Geometry: final body of the model. Coordinates: model frame, mm. Round coordinates to 2 decimals unless told otherwise and drop trailing zeros. Return JSON: item names as keys, results as strings. Group by question number.
Q1. Ray query, probe 1 along Y at (x, z) = (5.75, 0); probe 2 along Y at (x, z) = (5.5, -26.5); probe 3 along Z at (x, y) = (6.75, -94). Return the intervals inside material, ascending.
Q2. Mould query, pull axis Y, two halves, no side actions, for faces 1 (the face through (8, -32, 2)), 2 (the face through (4.06, 44.86, 39.25)), 3 (the face through (3.948, 154.672, 20.308)). Classes: released by +Y, released by -Y, zero draft, split by the parting line, or undercut.
Q3. Cut plane A-A on x = 4.25. Count the separate pieces of the cut face and the enclosed holes in it, and give its area (3 significant figures).
Q4. Contact query for flat-ended pins moving along their axis: pin 1 (6.5 mm diameter, centred on y = 42.43, z = 42.43, fed in from +X); pin 2 (3 mm diameter, centred on x = 3, y = 50, fed in from -Z); pin 3 (1 mm diameter, centred on x = 4.5, z = -58.5, fed in from +Y); pin 4 (3 mm diameter, centred on x = 7, z = 45, fed in from +Y). Output: stop coordinate, or through.
```python
from build123d import *

# Parameters (mm, degrees)
SKETCH_1_R               = 156
EXTRUDE_1_DEPTH          = 8
SKETCH_2_R               = 31
CUT_EXTRUDE_1_DEPTH      = 10
SKETCH_4_R               = 6
CUT_EXTRUDE_3_DEPTH      = 10
PATTERN_CIRCULAR_2_COUNT = 4
SKETCH_6_R               = 2
CUT_EXTRUDE_5_DEPTH      = 10
PATTERN_CIRCULAR_4_COUNT = 4
FILLET_1_R               = 0.3
SKETCH_8_R               = 4
CUT_EXTRUDE_7_DEPTH      = 10
SKETCH_9_R               = 30
CUT_EXTRUDE_8_DEPTH      = 10
PATTERN_CIRCULAR_6_COUNT = 4
PATTERN_CIRCULAR_7_COUNT = 2


with BuildPart() as part:
    # 草图1 → 凸台-拉伸1 (new body)
    with BuildSketch(Plane(origin=(0, 0, 0), x_dir=(0, 0, -1), z_dir=(1, 0, 0))):
        Circle(SKETCH_1_R)
    extrude(amount=EXTRUDE_1_DEPTH)

    # 草图2 → 切除-拉伸1 (cut)
    with BuildSketch(Plane(origin=(8, 0, 0), x_dir=(0, 0, -1), z_dir=(1, 0, 0))):
        Circle(SKETCH_2_R)
    extrude(amount=-CUT_EXTRUDE_1_DEPTH, mode=Mode.SUBTRACT)

    # 草图4 → 切除-拉伸3 (cut)
    with BuildSketch(Plane(origin=(8, 0, 0), x_dir=(0, 0, -1), z_dir=(1, 0, 0))):
        with Locations((91.923881554, 91.923881554)):
            Circle(SKETCH_4_R)
    cut_extrude_3 = extrude(amount=-CUT_EXTRUDE_3_DEPTH, mode=Mode.SUBTRACT)

    # 阵列(圆周)2: 切除-拉伸3 ×4 about axis
    pattern_circular_2_axis = Axis((0, 0, 0), (1, 0, 0))
    for i in range(1, PATTERN_CIRCULAR_2_COUNT):
        add(cut_extrude_3.rotate(pattern_circular_2_axis, i * 360 / PATTERN_CIRCULAR_2_COUNT), mode=Mode.SUBTRACT)

    # 草图6 → 切除-拉伸5 (cut)
    with BuildSketch(Plane(origin=(8, 0, 0), x_dir=(0, 0, -1), z_dir=(1, 0, 0))):
        with Locations((0, 36)):
            Circle(SKETCH_6_R)
    cut_extrude_5 = extrude(amount=-CUT_EXTRUDE_5_DEPTH, mode=Mode.SUBTRACT)

    # 阵列(圆周)4: 切除-拉伸5 ×4 about axis
    pattern_circular_4_axis = Axis((0, 0, 0), (1, 0, 0))
    for i in range(1, PATTERN_CIRCULAR_4_COUNT):
        add(cut_extrude_5.rotate(pattern_circular_4_axis, i * 360 / PATTERN_CIRCULAR_4_COUNT), mode=Mode.SUBTRACT)

    # 圆角1
    fillet_1_edges = [part.edges().sort_by_distance(p)[0] for p in [
        (0, 0, 156),
        (8, 0, 156),
    ]]
    fillet(fillet_1_edges, radius=FILLET_1_R)

    # 草图8 → 切除-拉伸7 (cut)
    with BuildSketch(Plane(origin=(8, 0, 0), x_dir=(0, 0, -1), z_dir=(1, 0, 0))):
        with Locations((42.426406871, -42.426406871)):
            Circle(SKETCH_8_R)
    cut_extrude_7 = extrude(amount=-CUT_EXTRUDE_7_DEPTH, mode=Mode.SUBTRACT)

    # 草图9 → 切除-拉伸8 (cut)
    with BuildSketch(Plane(origin=(8, 0, 0), x_dir=(0, 0, -1), z_dir=(1, 0, 0))):
        with Locations((0, 90)):
            Circle(SKETCH_9_R)
    cut_extrude_8 = extrude(amount=-CUT_EXTRUDE_8_DEPTH, mode=Mode.SUBTRACT)

    # 阵列(圆周)6: 切除-拉伸8 ×4 about axis
    pattern_circular_6_axis = Axis((0, 0, 0), (1, 0, 0))
    for i in range(1, PATTERN_CIRCULAR_6_COUNT):
        add(cut_extrude_8.rotate(pattern_circular_6_axis, i * 360 / PATTERN_CIRCULAR_6_COUNT), mode=Mode.SUBTRACT)

    # 阵列(圆周)7: 切除-拉伸7 ×2 about axis
    pattern_circular_7_axis = Axis((0, 0, 0), (1, 0, 0))
    for i in range(1, PATTERN_CIRCULAR_7_COUNT):
        add(cut_extrude_7.rotate(pattern_circular_7_axis, i * 360 / PATTERN_CIRCULAR_7_COUNT), mode=Mode.SUBTRACT)


solid = part.part
```
Result sheet:
{
 "1": {"probe 1": "y = -156 to -120, -60 to -38, -34 to -31, 31 to 34, 38 to 60, 120 to 156", "probe 2": "y = -153.73 to -104.06, -75.94 to -16.09, 16.09 to 75.94, 104.06 to 153.73", "probe 3": "z = -124.5 to -97.55, -86.29 to -29.73, 29.73 to 86.29, 97.55 to 124.5"},
 "2": {"face 1": "zero draft", "face 2": "undercut", "face 3": "split by the parting line"},
 "3": {"separate pieces": "1", "enclosed holes": "15", "area": "61,500 mm²"},
 "4": {"pin 1": "passes through", "pin 2": "stops at z = -148.27", "pin 3": "stops at y = 144.82", "pin 4": "stops at y = 149.81"}
}
